Part model, mm, in its own coordinate system. A direction names the side the tool comes from. Round coordinates to 2 decimals unless told otherwise and drop trailing zeros. Write each loop counter-clockwise with the first axis right and the second up, starting at its lowest first coordinate (ties: lowest second). Pieces come first, ordered by that corner, then holes. Notation, with made-up numbers: M -33.5,-29.75 L -7.5,-29.75 A36 cw -7.5,8.25 Z; hole C -9.5,30.5 d5. An arc over 180 degrees is marked long. Answer as a JSON object with one key per item and string values. Group by question number.
1. Drill centre lines: line 1 (Z direction, x = 5, y = 7); line 2 (X direction, y = 7.55, z = 7.5); line 3 (X direction, y = 7, z = -8). Where is each one in solid material? Low to high. Write a range as from..to.
2. Which spindle directions (+Z, -Z, +X, -X, +Y, -Y) get a long thin tool onto all of the face, cutting with end or side? Do faces 5 (the face through (-12, 6, 9.8)), 6 (the face through (-4.529, 8.028, 8.636)), 7 (the face through (12, 6, -9.8)). Say none if no direction does.
3. Band-saw the part on D-D, the plane y = 4. Write the cut outline in (x, z), plus the area to 3 significant figures.
4. Two-plate mould, pull along Z, no slides. Class faces 1 (the face through (-15, 7, 0)), 2 (the face through (-12, 6, -9.8)), 3 (the face through (-5.009, 5.39, 7.287)), 4 (the face through (5.471, 8.028, -6.364)): +Z half, -Z half, draft (parallel to the pull), parting line (faces both ways), or undercut.
5. Band-saw the part on B-B, the plane z = -1.75. Write the cut outline in (x, y).
6. Band-saw the part on A-A, the plane y = 9. Write the cut outline in (x, z), plus the area to 3 significant figures.
7. Drop flat-ended pins along their axis: pin 1 (3 mm diameter, centred on x = 13, y = 5.5, fed in from -Z); pin 2 (1.6 mm diameter, centred on x = -12.5, z = 4.5, fed in from +Y); pin 3 (2 mm diameter, centred on x = -5, z = -7.5, fed in from +Y). Give the stop position or say it passes through.
from build123d import *

# Parameters (mm, degrees)
SKETCH1_W               = 19.6
SKETCH1_H               = 7.5
BOSS_EXTRUDE1_DEPTH     = 15
SKETCH2_W               = 20
SKETCH2_H               = 7.8
BOSS_EXTRUDE2_DEPTH     = 9.5
CUT_EXTRUDE2_DEPTH      = 21.615528128
CUT_EXTRUDE2_DEPTH_BACK = 21.615528128
CHAMFER1_SIZE           = 0.3
CHAMFER2_SIZE           = 0.3
CHAMFER3_SIZE           = 0.3
CHAMFER4_SIZE           = 0.3
LPATTERN2_COUNT         = 2
LPATTERN2_PITCH         = 10
LPATTERN2_COUNT_DIR2    = 2
LPATTERN2_PITCH_DIR2    = 15


with BuildPart() as part:
    # Sketch1 → Boss-Extrude1 (new, symmetric)
    with BuildSketch(Plane(origin=(0, 0, 0), x_dir=(0, 0, -1), z_dir=(1, 0, 0))):
        with Locations((0, 5.95)):
            Rectangle(SKETCH1_W, SKETCH1_H)
    extrude(amount=BOSS_EXTRUDE1_DEPTH, both=True)

    # Sketch2 → Boss-Extrude2 (add, symmetric)
    with BuildSketch(Plane(origin=(0, 0, 0), x_dir=(0, 0, -1), z_dir=(1, 0, 0))):
        with Locations((0, 6.1)):
            Rectangle(SKETCH2_W, SKETCH2_H)
    extrude(amount=BOSS_EXTRUDE2_DEPTH, both=True)

    # Sketch4 → Cut-Extrude2 (cut, two sides: drawn at the far end of the back side and taken through both)
    with BuildSketch(Plane(origin=(0, 0, 0), x_dir=(0, 0, -1), z_dir=(1, 0, 0)).offset(-CUT_EXTRUDE2_DEPTH_BACK)):
        with BuildLine():
            Line((-4.3, 5.5), (4.3, 5.5))
            Line((4.3, 5.5), (4.5, 5.3))
            Line((4.5, 5.3), (4.5, 5.04428602))
            Line((4.5, 5.04428602), (4.22, 4.882627944))
            ThreePointArc((4.22, 4.882627944), (3.942636741, 4.654893122), (3.753338798, 4.35))
            Line((3.753338798, 4.35), (3.1, 4.35))
            Line((3.1, 4.35), (3.1, 3.65))
            Line((3.1, 3.65), (3.753338798, 3.65))
            ThreePointArc((3.753338798, 3.65), (3.942636741, 3.345106878), (4.22, 3.117372056))
            Line((4.22, 3.117372056), (4.5, 2.95571398))
            Line((4.5, 2.95571398), (4.5, 0))
            Line((4.5, 0), (-4.5, 0))
            Line((-4.5, 0), (-4.5, 2.95571398))
            Line((-4.5, 2.95571398), (-4.22, 3.117372056))
            ThreePointArc((-4.22, 3.117372056), (-3.942636741, 3.345106878), (-3.753338798, 3.65))
            Line((-3.753338798, 3.65), (-3.1, 3.65))
            Line((-3.1, 3.65), (-3.1, 4.35))
            Line((-3.1, 4.35), (-3.753338798, 4.35))
            ThreePointArc((-3.753338798, 4.35), (-3.942636741, 4.654893122), (-4.22, 4.882627944))
            Line((-4.22, 4.882627944), (-4.5, 5.04428602))
            Line((-4.5, 5.04428602), (-4.5, 5.3))
            Line((-4.5, 5.3), (-4.3, 5.5))
        make_face()
    extrude(amount=CUT_EXTRUDE2_DEPTH + CUT_EXTRUDE2_DEPTH_BACK, mode=Mode.SUBTRACT)

    # Chamfer1
    chamfer1_edges = [part.edges().sort_by_distance(p)[0] for p in [
        (-12.25, 9.7, 9.8),
        (-12.25, 9.7, -9.8),
        (12.25, 9.7, 9.8),
        (12.25, 9.7, -9.8),
    ]]
    chamfer(chamfer1_edges, length=CHAMFER1_SIZE)

    # Chamfer2
    chamfer2_edges = [part.edges().sort_by_distance(p)[0] for p in [
        (0, 10, 10),
        (0, 10, -10),
    ]]
    chamfer(chamfer2_edges, length=CHAMFER2_SIZE)

    # Chamfer3
    chamfer3_edges = [part.edges().sort_by_distance(p)[0] for p in [
        (-12.25, 2.2, -9.8),
        (-12.25, 2.2, 9.8),
        (12.25, 2.2, -9.8),
        (12.25, 2.2, 9.8),
    ]]
    chamfer(chamfer3_edges, length=CHAMFER3_SIZE)

    # Chamfer4
    chamfer4_edges = [part.edges().sort_by_distance(p)[0] for p in [
        (0, 2.2, 10),
        (0, 2.2, -10),
    ]]
    chamfer(chamfer4_edges, length=CHAMFER4_SIZE)

    # Sketch7 → Tap2 (revolve, cut)
    with BuildSketch(Plane(origin=(-5, 10, -7.5), x_dir=(0, 0, 1), z_dir=(1, 0, 0))):
        Polygon((0, 0), (0, 4.738758131), (1.2295, 4), (1.2295, 0), align=None)
    tap2 = revolve(axis=Axis((-5, 10, -7.5), (0, -1, 0)), mode=Mode.SUBTRACT)

    # LPattern2: Tap2 2 × 2
    with Locations(*[(i * LPATTERN2_PITCH, 0, j * LPATTERN2_PITCH_DIR2) for i in range(LPATTERN2_COUNT) for j in range(LPATTERN2_COUNT_DIR2) if (i, j) != (0, 0)]):
        add(tap2, mode=Mode.SUBTRACT)


solid = part.part
Worked answers:
{
 "1": {"line 1": "z = -10..-8.73, -6.27..6.27, 8.73..10", "line 2": "x = -15..-6.23, -3.77..3.77, 6.23..15", "line 3": "x = -15..-6.12, -3.88..3.88, 6.12..15"},
 "2": {"face 5": "+Z, -X, +Y, -Y", "face 6": "+Y", "face 7": "-Z, +X, +Y, -Y"},
 "3": {"outline": "M -15,-9.8 L -9.5,-9.8 L -9.5,-10 L 9.5,-10 L 9.5,-9.8 L 15,-9.8 L 15,-3.1 L -15,-3.1 Z; M -15,3.1 L 15,3.1 L 15,9.8 L 9.5,9.8 L 9.5,10 L -9.5,10 L -9.5,9.8 L -15,9.8 Z", "area": "410 mm^2"},
 "4": {"face 1": "draft", "face 2": "-Z half", "face 3": "undercut", "face 4": "undercut"},
 "5": {"outline": "M -15,5.5 L 15,5.5 L 15,9.7 L 9.5,9.7 L 9.5,10 L -9.5,10 L -9.5,9.7 L -15,9.7 Z"},
 "6": {"outline": "M -15,-9.8 L -9.5,-9.8 L -9.5,-10 L 9.5,-10 L 9.5,-9.8 L 15,-9.8 L 15,9.8 L 9.5,9.8 L 9.5,10 L -9.5,10 L -9.5,9.8 L -15,9.8 Z; hole C -5,-7.5 d2.46; hole C -5,7.5 d2.46; hole C 5,-7.5 d2.46; hole C 5,7.5 d2.46", "area": "577 mm^2"},
 "7": {"pin 1": "stops at z = -9.8", "pin 2": "stops at y = 9.7", "pin 3": "stops at y = 5.86"}
}
